Can you work these out from the model? Positions are in its coordinate system, mm. A direction names the side the tool comes from. Round coordinates to 2 decimals unless told otherwise and drop trailing zeros. Loops run counter-clockwise (first coordinate to the right, second up) from the corner with the lowest first, then second, coordinate; pieces in that order, holes last.
```python
from build123d import *

# Parameters (mm, degrees)
SKETCH005_W             = 80
SKETCH005_H             = 20
SKETCH005_R             = 2.75
PAD010_DEPTH            = 8
POCKET009_DEPTH         = 4
SKETCH011_W             = 24.5
SKETCH011_H             = 2.666667
POCKET010_DEPTH         = 185.699521
SKETCH017_R             = 2.25
PAD011_DEPTH            = 4
BODY002_PLACEMENT_ANGLE = 180


with BuildPart() as part:
    # Sketch005 → Pad010 (new body)
    with BuildSketch(Plane.XZ):
        Rectangle(SKETCH005_W, SKETCH005_H)
        Circle(SKETCH005_R, mode=Mode.SUBTRACT)
    extrude(amount=PAD010_DEPTH)

    # Sketch007 → Pocket009 (cut)
    with BuildSketch(Plane.XZ.offset(8)):
        Polygon((4.113621, 2.375), (0, 4.75), (-4.113621, 2.375), (-4.113621, -2.375), (0, -4.75), (4.113621, -2.375), align=None)
    extrude(amount=-POCKET009_DEPTH, mode=Mode.SUBTRACT)

    # Sketch011 → Pocket010 (cut, through all)
    with BuildSketch(Plane(origin=(0, 0, 10), x_dir=(-1, 0, 0), z_dir=(0, 0, 1))):
        with Locations((-21.75, 4.333334)):
            Rectangle(SKETCH011_W, SKETCH011_H)
    pocket010 = extrude(amount=-POCKET010_DEPTH, mode=Mode.SUBTRACT)

    # Sketch017 (on Face4 of Pad010) → Pad011 (join)
    with BuildSketch(Plane(origin=(-40, 0, 0), x_dir=(0, 0, -1), z_dir=(-1, 0, 0))):
        with BuildLine():
            Line((-10, 0), (10, 0))
            Line((10, 0), (10, 35.5))
            ThreePointArc((10, 35.5), (0, 45.5), (-10, 35.5))
            Line((-10, 35.5), (-10, 0))
        make_face()
        with Locations((0, 40)):
            Circle(SKETCH017_R, mode=Mode.SUBTRACT)
    pad011 = extrude(amount=PAD011_DEPTH)

    # Mirrored007: Pad011 across YZ
    add(pad011.mirror(Plane.YZ))

    # Mirrored008: Pocket010 across YZ
    add(pocket010.mirror(Plane.YZ), mode=Mode.SUBTRACT)


with BuildPart() as part_1:
    # Body002 placement: moved
    add(part.part.moved(Location((0, 2, 9))).rotate(Axis((0, 2, 9), (1, 0, 0)), BODY002_PLACEMENT_ANGLE))


solid = part_1.part
```
(1) Which directions (+Z, -Z, +X, -X, +Y, -Y) give clear straight access to the entire face, cutting with the end or side of a thin tool? Please do faces 1 (the flat face through (2.03, 8.03, 12.58)), 2 (the flat face through (-9.5, 6, 9)), 3 (the flat face through (-1, 10, 4)).
(2) Suppose I cut it at C-C (x = -17.5). Write out the boundary of the cut face in (y, z).
(3) Suppose I cut it at A-A (z = 9). Give the number of separate pieces and of enclosed holes in the cut face, then the cut area to 3 significant figures.
(4) Suppose I cut it at D-D (z = 3). Write out the boundary of the cut face in (x, y), then the cut area to 3 significant figures.
(5) For pin 1 (6.5 mm diameter, centred on x = -1, z = 7.5, fed in from +Y); pin 2 (4 mm diameter, centred on y = 42, z = 9, fed in from +X), each with a flat end and sliding along its axis, tell me the tip position at first contact or that it passes through.
(6) We'd pull the mould along X, two halves only. Please class faces 4 (the flat face through (44, 25, 9)), 5 (the flat face through (22, 5, 9)), 6 (the flat face through (-1, 2, 13)): released by +X, released by -X, zero draft, split by the parting line, or undercut.
(7) Suppose I cut it at B-B (y = 34). Write out the boundary of the cut face in (x, z), then the cut area to 3 significant figures.
(8) If I drill on line 1 (X direction, y = 42, z = 2.5); line 2 (Y direction, x = 41.8, z = 9); line 3 (Y direction, x = 14.5, z = 8.5), over which ranges is the centre line in solid material (lowest first)?
Check result:
1. face 1: +Y
1. face 2: +Z, -Z
1. face 3: +Z, -Z, +Y
2. outline: (2, -1) - (5, -1) - (5, 19) - (2, 19) - close; (7.67, -1) - (10, -1) - (10, 19) - (7.67, 19) - close
3. separate pieces: 4
3. enclosed holes: 2
3. area: 782 mm2
4. outline: (-44, 2) - (44, 2) - (44, 45.5) - (40, 45.5) - (40, 10) - (-40, 10) - (-40, 45.5) - (-44, 45.5) - close; hole (-34, 5) - (-9.5, 5) - (-9.5, 7.67) - (-34, 7.67) - close; hole (9.5, 5) - (34, 5) - (34, 7.67) - (9.5, 7.67) - close
4. area: 857 mm2
5. pin 1: stops at y = 10
5. pin 2: passes through
6. face 4: released by +X
6. face 5: undercut
6. face 6: zero draft
7. outline: (-44, -1) - (-40, -1) - (-40, 19) - (-44, 19) - close; (40, -1) - (44, -1) - (44, 19) - (40, 19) - close
7. area: 160 mm2
8. line 1: x = -44 to -40, 40 to 44
8. line 2: y = 2 to 39.75, 44.25 to 47.5
8. line 3: y = 2 to 5, 7.67 to 10
